The model under review builds one solid part; all positions refer to its coordinate system, in mm. A direction names the side the tool comes from. Give positions to 0.01 mm unless a question says otherwise; leave off trailing zeros. Order: outer loops, then holes, each group sorted by start corner. A loop starts at its lowest first (then second) coordinate and runs counter-clockwise, first axis right, second up. Notation, with made-up numbers: (27, -5.75) - (79, -5.75) arc R29 ccw to (79, 33.25) - close; hole circle Ø9 at (46, -34). An arc over 180 degrees is marked (long way). Put each result on its own line as item: value.
```python
from build123d import *

# Parameters (mm, degrees)
SKETCH2_R          = 50
CUT_EXTRUDE1_DEPTH = 828.647267862


with BuildPart() as part:
    # Sketch1 → Revolve1 (revolve)
    with BuildSketch(Plane(origin=(0, 0, 0), x_dir=(0, 0, -1), z_dir=(1, 0, 0)), mode=Mode.PRIVATE) as revolve1_sk:
        Polygon((0, 0), (0, 250), (450, 250), (450, 0), (350, 0), (350, -100), (300, -100), (300, 0), (150, 0), (150, -100), (100, -100), (100, 0), align=None)
    revolve(revolve1_sk.sketch.rotate(Axis((0, 250, 0), (0, 0, -1)), 270), axis=Axis((0, 250, 0), (0, 0, -1)))

    # Sketch2 → Cut-Extrude1 (cut, through all)
    with BuildSketch(Plane(origin=(0, 0, -450), x_dir=(-1, 0, 0), z_dir=(0, 0, -1))):
        with Locations((0, 250)):
            Circle(SKETCH2_R)
    extrude(amount=-CUT_EXTRUDE1_DEPTH, mode=Mode.SUBTRACT)


solid = part.part
```
(1) Take a section at C-C, the plane z = -394. Write out the cut boundary in (x, y).
The answers:
outline: circle Ø500 at (0, 250); hole circle Ø100 at (0, 250)
(2) Wall thickness on L1, parallel to Y at x = 0, z = -253.5; L2, parallel to Z at x = -107, y = -37; L3, parallel to Y at x = 0, z = -329: over which ranges is each line inside the solid? List them lowest first.
The answers:
L1: 0 to 200, 300 to 500
L2: -350 to -300, -150 to -100
L3: -100 to 200, 300 to 600
(3) For faces 4 (the flat face through (83, 12, -350)), 5 (the cylindrical face through (-277.75, 462.97, -124.65)), 6 (the flat face through (-3, 302, 0)), 7 (the cylindrical face through (-32.55, 2.13, -49.3)), 8 (the cylindrical face through (-32.55, 2.13, -223.95)), list the 3-axis set-ups (+Z, -Z, +X, -X, +Y, -Y) from which the entire face can be reached by the end or side of a thin tool; tool diameter is ignored.
The answers:
face 4: -Z
face 5: +Z, -Z
face 6: +Z, +X, -X, +Y, -Y
face 7: +Z
face 8: none
(4) Clearance check with flat-ended pins moving along their axes: pin 1 Ø1.5 at (y, z) = (187, -92.5) entering from -X; pin 2 Ø8 at (x, z) = (165.5, -394) entering from +Y; pin 3 Ø2 at (y, z) = (34, -222) entering from -X. State where each tip first meets the part, or that it passes through.
The answers:
pin 1: x = -242.13
pin 2: y = 440.83
pin 3: x = -127.57
(5) The part is to be moulded in two halves that separate along X. For faces 1 (the flat face through (3, 302, -450)), 2 (the cylindrical face through (-32.55, 2.13, -399.3)), 3 (the cylindrical face through (6.509, 299.575, -228.15)), say which applies: pulls with the +X half, pulls with the -X half, needs draft (parallel to the pull), parting line crosses it, or undercut.
The answers:
face 1: needs draft
face 2: parting line crosses it
face 3: undercut
(6) Take a section at D-D, the plane x = 207.5. Write out the cut boundary in (y, z).
The answers:
outline: (-31.86, -350) - (110.56, -350) - (110.56, -450) - (389.44, -450) - (389.44, -350) - (531.86, -350) - (531.86, -300) - (389.44, -300) - (389.44, -150) - (531.86, -150) - (531.86, -100) - (389.44, -100) - (389.44, 0) - (110.56, 0) - (110.56, -100) - (-31.86, -100) - (-31.86, -150) - (110.56, -150) - (110.56, -300) - (-31.86, -300) - close
(7) Take a section at B-B, the plane x = 0. Write out the cut boundary in (y, z), then the cut area to 3 significant figures.
The answers:
outline: (-100, -350) - (0, -350) - (0, -450) - (200, -450) - (200, 0) - (0, 0) - (0, -100) - (-100, -100) - (-100, -150) - (0, -150) - (0, -300) - (-100, -300) - close; (300, -450) - (500, -450) - (500, -350) - (600, -350) - (600, -300) - (500, -300) - (500, -150) - (600, -150) - (600, -100) - (500, -100) - (500, 0) - (300, 0) - close
area: 200,000 mm^2
(8) Take a section at A-A, the plane y = 250. Write out the cut boundary in (x, z).
The answers:
outline: (-350, -350) - (-250, -350) - (-250, -450) - (-50, -450) - (-50, 0) - (-250, 0) - (-250, -100) - (-350, -100) - (-350, -150) - (-250, -150) - (-250, -300) - (-350, -300) - close; (50, -450) - (250, -450) - (250, -350) - (350, -350) - (350, -300) - (250, -300) - (250, -150) - (350, -150) - (350, -100) - (250, -100) - (250, 0) - (50, 0) - close
